Input: part model. Units: mm. Frame: model coordinates. A direction names the side the tool comes from. Give positions to 0.01 mm unless a question says otherwise; leave off trailing zeros. Loops run counter-clockwise (first coordinate to the right, second up) from the corner with the lowest first, then second, coordinate; pieces in that order, holes last.
from build123d import *

# Parameters (mm, degrees)
SKETCH_1_W          = 120
SKETCH_1_H          = 120
EXTRUDE_1_DEPTH     = 100
SKETCH_2_R          = 47.5
CUT_EXTRUDE_1_DEPTH = 10
SKETCH_3_R          = 45
CUT_EXTRUDE_2_DEPTH = 17.5
SKETCH_4_W          = 120
SKETCH_4_H          = 120
CUT_EXTRUDE_3_DEPTH = 49.5
SKETCH_6_W          = 120
SKETCH_6_H          = 120
CUT_EXTRUDE_5_DEPTH = 13
CUT_EXTRUDE_6_DEPTH = 13
SKETCH_8_R          = 2.25
CUT_EXTRUDE_7_DEPTH = 13
SKETCH_10_R         = 2.25
CUT_EXTRUDE_8_DEPTH = 13
FILLET_1_R          = 20
FILLET_2_R          = 20
SKETCH_11_R         = 1.5
CUT_EXTRUDE_9_DEPTH = 10
EXTRUDE_START       = 40
EXTRUDE_3_DEPTH     = 40


with BuildPart() as part:
    # 草图1 → 凸台-拉伸1 (new body)
    with BuildSketch(Plane.XY):
        Rectangle(SKETCH_1_W, SKETCH_1_H)
    extrude(amount=EXTRUDE_1_DEPTH)

    # 草图2 → 切除-拉伸1 (cut)
    with BuildSketch(Plane(origin=(0, 0, 0), x_dir=(-1, 0, 0), z_dir=(0, 0, -1))):
        Circle(SKETCH_2_R)
    extrude(amount=-CUT_EXTRUDE_1_DEPTH, mode=Mode.SUBTRACT)

    # 草图3 → 切除-拉伸2 (cut)
    with BuildSketch(Plane(origin=(0, 0, 10), x_dir=(-1, 0, 0), z_dir=(0, 0, -1))):
        Circle(SKETCH_3_R)
    extrude(amount=-CUT_EXTRUDE_2_DEPTH, mode=Mode.SUBTRACT)

    # 草图4 → 切除-拉伸3 (cut)
    with BuildSketch(Plane.XY.offset(100)):
        Rectangle(SKETCH_4_W, SKETCH_4_H)
    extrude(amount=-CUT_EXTRUDE_3_DEPTH, mode=Mode.SUBTRACT)

    # 草图6 → 切除-拉伸5 (cut)
    with BuildSketch(Plane.XY.offset(50.5)):
        Rectangle(SKETCH_6_W, SKETCH_6_H)
    extrude(amount=-CUT_EXTRUDE_5_DEPTH, mode=Mode.SUBTRACT)

    # 草图7 → 切除-拉伸6 (cut)
    with BuildSketch(Plane(origin=(0, 0, 27.5), x_dir=(-1, 0, 0), z_dir=(0, 0, -1))):
        Polygon((-10, 10), (30, 10), (30, -10), (-10, -10), (-10, 0), align=None)
    extrude(amount=-CUT_EXTRUDE_6_DEPTH, mode=Mode.SUBTRACT)

    # 草图8 → 切除-拉伸7 (cut)
    with BuildSketch(Plane(origin=(0, 0, 27.5), x_dir=(-1, 0, 0), z_dir=(0, 0, -1))):
        with Locations((-14, 5.1)):
            Circle(SKETCH_8_R)
        with Locations((-14, -5.1)):
            Circle(SKETCH_8_R)
    extrude(amount=-CUT_EXTRUDE_7_DEPTH, mode=Mode.SUBTRACT)

    # 草图10 → 切除-拉伸8 (cut)
    with BuildSketch(Plane(origin=(0, 0, 27.5), x_dir=(-1, 0, 0), z_dir=(0, 0, -1))):
        with Locations((34, 5.1)):
            Circle(SKETCH_10_R)
        with Locations((34, -5.1)):
            Circle(SKETCH_10_R)
    extrude(amount=-CUT_EXTRUDE_8_DEPTH, mode=Mode.SUBTRACT)

    # 圆角1
    fillet_1_edges = [part.edges().sort_by_distance(p)[0] for p in [
        (60, 60, 18.75),
    ]]
    fillet(fillet_1_edges, radius=FILLET_1_R)

    # 圆角2
    fillet_2_edges = [part.edges().sort_by_distance(p)[0] for p in [
        (60, -60, 18.75),
        (-60, -60, 18.75),
        (-60, 60, 18.75),
    ]]
    fillet(fillet_2_edges, radius=FILLET_2_R)

    # 草图11 → 切除-拉伸9 (cut)
    with BuildSketch(Plane(origin=(0, 0, 0), x_dir=(-1, 0, 0), z_dir=(0, 0, -1))):
        with Locations((-38.890872965, 38.890872965)):
            Circle(SKETCH_11_R)
        with Locations((38.890872965, 38.890872965)):
            Circle(SKETCH_11_R)
        with Locations((38.890872965, -38.890872965)):
            Circle(SKETCH_11_R)
        with Locations((-38.890872965, -38.890872965)):
            Circle(SKETCH_11_R)
    extrude(amount=-CUT_EXTRUDE_9_DEPTH, mode=Mode.SUBTRACT)

    # 草图12 → 凸台-拉伸3 (add)
    with BuildSketch(Plane.XY.offset(37.5).offset(EXTRUDE_START)):
        with BuildLine():
            Line((-40, 40), (-40, 60))
            ThreePointArc((-40, 60), (-54.142135624, 54.142135624), (-60, 40))
            Line((-60, 40), (-40, 40))
        make_face()
        with BuildLine():
            Line((40, 40), (40, 60))
            ThreePointArc((40, 60), (54.142135624, 54.142135624), (60, 40))
            Line((60, 40), (40, 40))
        make_face()
        with BuildLine():
            Line((40, -40), (60, -40))
            ThreePointArc((60, -40), (54.142135624, -54.142135624), (40, -60))
            Line((40, -60), (40, -40))
        make_face()
        with BuildLine():
            Line((-40, -40), (-40, -60))
            ThreePointArc((-40, -60), (-54.142135624, -54.142135624), (-60, -40))
            Line((-60, -40), (-40, -40))
        make_face()
    extrude(amount=-EXTRUDE_3_DEPTH)


solid = part.part
(1) Reachability of faces 4 (the flat face through (10, 0, 32)), 5 (the flat face through (50, -40, 58)), 6 (the flat face through (39, -39, 10)), 7 (the flat face through (48, -48, 77.5)), 8 (the flat face through (-28, 41, 0)) from +Z, -Z, +X, -X, +Y, -Y: full face, straight path, thin tool, end or side. Return the list, or none.
Values follow:
face 4: +Z, -Z
face 5: +Z, +X, -X
face 6: -Z
face 7: +Z, +X, -X, +Y, -Y
face 8: -Z, +X, -X, +Y, -Y
(2) Pin query (flat end, axial travel): pin 1 Ø3.5 at (x, y) = (38.89, -38.89) entering from -Z; pin 2 Ø5 at (x, y) = (14, -5.1) entering from -Z; pin 3 Ø6 at (x, z) = (-45.5, 57.5) entering from +Y; pin 4 Ø10 at (x, z) = (47.5, 51.5) entering from -Y. Return the tip coordinate at first contact, or that it passes through.
Values follow:
pin 1: stops at z = 0
pin 2: stops at z = 27.5
pin 3: stops at y = 59.84
pin 4: stops at y = -59.84
(3) Cut plane B-B (x = 0). Return the cut outline in (y, z), and give its area (4 significant figures).
Values follow:
outline: (-60, 0) - (-47.5, 0) - (-47.5, 10) - (-45, 10) - (-45, 27.5) - (-10, 27.5) - (-10, 37.5) - (-60, 37.5) - close; (10, 27.5) - (45, 27.5) - (45, 10) - (47.5, 10) - (47.5, 0) - (60, 0) - (60, 37.5) - (10, 37.5) - close
area: 1,775 mm2
(4) Cut plane A-A (y = 0). Return the cut outline in (x, z), and give its area (4 significant figures).
Values follow:
outline: (-60, 0) - (-47.5, 0) - (-47.5, 10) - (-45, 10) - (-45, 27.5) - (-30, 27.5) - (-30, 37.5) - (-60, 37.5) - close; (10, 27.5) - (45, 27.5) - (45, 10) - (47.5, 10) - (47.5, 0) - (60, 0) - (60, 37.5) - (10, 37.5) - close
area: 1,575 mm2
(5) Ray query, probe 1 along Y at (x, z) = (-34, 32.25); probe 2 along Y at (x, z) = (0, 22.75); probe 3 along Z at (x, y) = (54, 30). Return the intervals inside material, ascending.
Values follow:
probe 1: y = -60 to -7.35, -2.85 to 2.85, 7.35 to 60
probe 2: y = -60 to -45, 45 to 60
probe 3: z = 0 to 37.5
(6) Cut plane C-C (z = 70). Return the cut outline in (x, y).
Values follow:
outline: (-60, -40) arc R20 ccw to (-40, -60) - (-40, -40) - close; (-60, 40) - (-40, 40) - (-40, 60) arc R20 ccw to start; (40, -60) arc R20 ccw to (60, -40) - (40, -40) - close; (40, 40) - (60, 40) arc R20 ccw to (40, 60) - close
(7) Mould query, pull axis X, two halves, no side actions, for faces 1 (the flat face through (48, 48, 77.5)), 2 (the cylindrical face through (-36.08, 4.24, 32.43)), 3 (the cylindrical face through (-40.32, -38.44, 4.93)). Classes: +X half, -X half, draft (parallel to the pull), parting line (faces both ways), or undercut.
Values follow:
face 1: draft
face 2: undercut
face 3: undercut
(8) Cut plane D-D (x = -34). Return the cut outline in (y, z), and give its area (3 significant figures).
Values follow:
outline: (-60, 0) - (-33.17, 0) - (-33.17, 10) - (-29.48, 10) - (-29.48, 27.5) - (-7.35, 27.5) - (-7.35, 37.5) - (-60, 37.5) - close; (-2.85, 27.5) - (2.85, 27.5) - (2.85, 37.5) - (-2.85, 37.5) - close; (7.35, 27.5) - (29.48, 27.5) - (29.48, 10) - (33.17, 10) - (33.17, 0) - (60, 0) - (60, 37.5) - (7.35, 37.5) - close
area: 2,710 mm2
